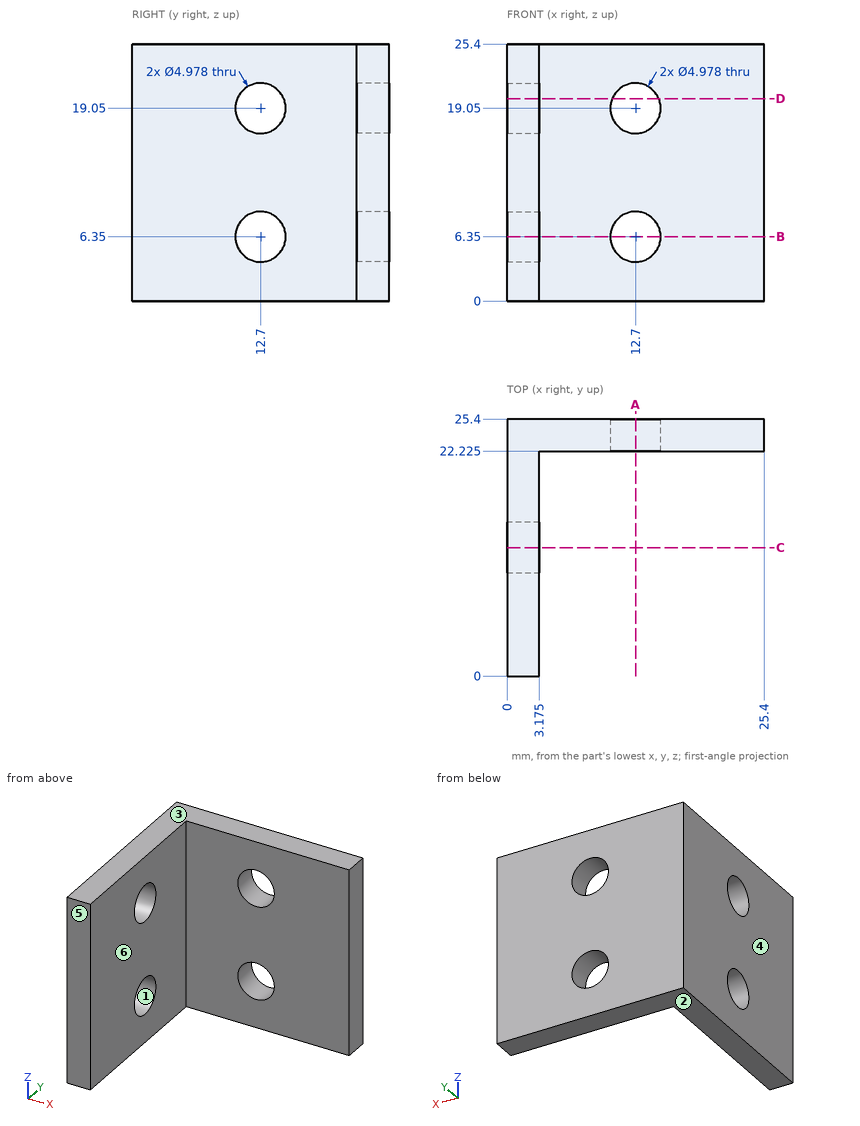
Input: dimensioned drawing with shaded views. Units: mm. Origin: part minimum x, y, z. A direction names the side the tool comes from. Give positions to 0.01 mm unless a question says otherwise; leave off trailing zeros. Loops run counter-clockwise (first coordinate to the right, second up) from the corner with the lowest first, then second, coordinate; pieces in that order, holes last. Notation, with made-up numbers: (65.25, -12) - (81.25, -12) arc R12 cw to (81.25, 2) - close; hole circle Ø1 at (71, 79). An arc over 180 degrees is marked (long way). Answer as CSV lines item,"result". Start each with the question number.
(1) Section query C-C (y = 12.7). Output: boundary loops of the cut face in (x, z) (1 decimal).
(2) Mould query, pull axis Z, two halves, no side actions, for the marked faces 1, 2, 3 and 4. Classes: +Z half, -Z half, draft (parallel to the pull), parting line (faces both ways), or undercut.
(3) Section query B-B (z = 6.35). Output: boundary loops of the cut face in (x, y) (1 decimal).
(4) Pin query (flat end, axial travel): P1, Ø4, axis at x = 12.7, z = 6.35, coming from the +Y side; P2, Ø6, axis at y = 16, z = 18, coming from the -X side; P3, Ø2, axis at y = 8, z = 21.5, coming from the +X side (3 decimals); P4, Ø6.5, axis at x = 14.5, z = 7.5, coming from the -Y side (3 decimals). Return the tip coordinate at first contact, or that it passes through.
(5) Reachability of the marked faces 5 and 6 from +Z, -Z, +X, -X, +Y, -Y: full face, straight path, thin tool, end or side. Return the list, or none.
(6) Section query A-A (x = 12.7). Output: boundary loops of the cut face in (y, z) (1 decimal).
(7) Ray query, line 1 along Z through (x, y) = (12.7, 24.4); line 2 along Y through (x, z) = (18, 21.5) (1 decimal); line 3 along X through (y, z) = (19.5, 18) (1 decimal). Return the intervals inside material, ascending. Write a range as [from, to].
(8) Section query D-D (z = 20). Output: boundary loops of the cut face in (x, y) (1 decimal).
Worked answers:
1,outline,"(0, 0) - (3.2, 0) - (3.2, 3.9) - (0, 3.9) - close; (0, 8.8) - (3.2, 8.8) - (3.2, 16.6) - (0, 16.6) - close; (0, 21.5) - (3.2, 21.5) - (3.2, 25.4) - (0, 25.4) - close"
2,face 1,"undercut"
2,face 2,"-Z half"
2,face 3,"+Z half"
2,face 4,"draft"
3,outline,"(0, 0) - (3.2, 0) - (3.2, 10.2) - (0, 10.2) - close; (0, 15.2) - (3.2, 15.2) - (3.2, 22.2) - (10.2, 22.2) - (10.2, 25.4) - (0, 25.4) - close; (15.2, 22.2) - (25.4, 22.2) - (25.4, 25.4) - (15.2, 25.4) - close"
4,P1,"passes through"
4,P2,"stops at x = 0"
4,P3,"stops at x = 3.175"
4,P4,"stops at y = 22.225"
5,face 5,"+Z, -Z, +X, -X, -Y"
5,face 6,"+Z, -Z, +X, -Y"
6,outline,"(22.2, 0) - (25.4, 0) - (25.4, 3.9) - (22.2, 3.9) - close; (22.2, 8.8) - (25.4, 8.8) - (25.4, 16.6) - (22.2, 16.6) - close; (22.2, 21.5) - (25.4, 21.5) - (25.4, 25.4) - (22.2, 25.4) - close"
7,line 1,"z = [0, 3.86], [8.84, 16.56], [21.54, 25.4]"
7,line 2,"y = [22.2, 25.4]"
7,line 3,"x = [0, 3.2]"
8,outline,"(0, 0) - (3.2, 0) - (3.2, 10.4) - (0, 10.4) - close; (0, 15) - (3.2, 15) - (3.2, 22.2) - (10.4, 22.2) - (10.4, 25.4) - (0, 25.4) - close; (15, 22.2) - (25.4, 22.2) - (25.4, 25.4) - (15, 25.4) - close"
